```python
from build123d import *

# Parameters (mm, degrees)
F0_R     = 20
F0_R_2   = 1.5
F1_DEPTH = 4
F2_R     = 21.4
F2_R_2   = 20
F3_DEPTH = 1
F4_R     = 21.4
F4_R_2   = 20
F5_DEPTH = 1


with BuildPart() as f1:
    # F0 (on Top) → F1 (new body)
    with BuildSketch(Plane.XY):
        Circle(F0_R)
        Circle(F0_R_2, mode=Mode.SUBTRACT)
    extrude(amount=F1_DEPTH)

    # F2 (on face) → F3 (join)
    with BuildSketch(Plane.XY.offset(4)):
        Circle(F2_R)
        Circle(F2_R_2, mode=Mode.SUBTRACT)
    extrude(amount=-F3_DEPTH)

    # F4 (on face) → F5 (join)
    with BuildSketch(Plane(origin=(0, 0, 0), x_dir=(1, 0, 0), z_dir=(0, 0, -1))):
        Circle(F4_R)
        Circle(F4_R_2, mode=Mode.SUBTRACT)
    extrude(amount=-F5_DEPTH)


solid = f1.part
```
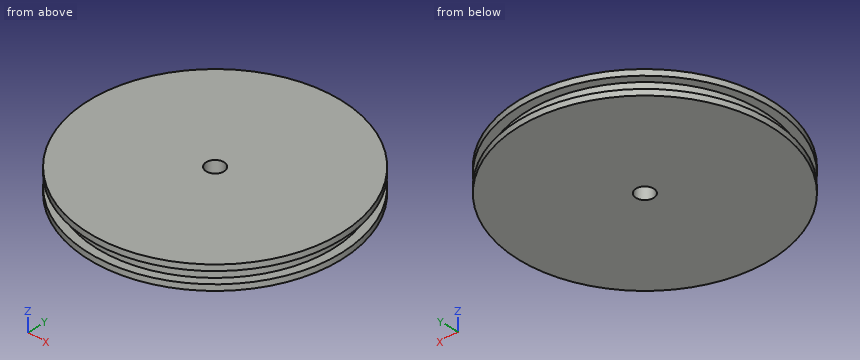
Input: part model. Units: mm. Frame: model coordinates. Give positions to 0.01 mm unless a question says otherwise; leave off trailing zeros. Order: outer loops, then holes, each group sorted by start corner. A loop starts at its lowest first (then second) coordinate and runs counter-clockwise, first axis right, second up.
1. Cut plane A-A (y = 0). Return loops of the section in (x, z), and give its area (3 significant figures).
Computed:
outline: (-21.4, 0) - (-1.5, 0) - (-1.5, 4) - (-21.4, 4) - (-21.4, 3) - (-20, 3) - (-20, 1) - (-21.4, 1) - close; (1.5, 0) - (21.4, 0) - (21.4, 1) - (20, 1) - (20, 3) - (21.4, 3) - (21.4, 4) - (1.5, 4) - close
area: 154 mm2
2. Cut plane C-C (x = -12.5). Return loops of the section in (y, z), and give its area (3 significant figures).
Computed:
outline: (-17.37, 0) - (17.37, 0) - (17.37, 1) - (15.61, 1) - (15.61, 3) - (17.37, 3) - (17.37, 4) - (-17.37, 4) - (-17.37, 3) - (-15.61, 3) - (-15.61, 1) - (-17.37, 1) - close
area: 132 mm2
3. Pin query (flat end, axial travel): pin 1 Ø13 at (x, y) = (-7, -1.5) entering from -Z; pin 2 Ø2 at (y, z) = (9.5, 2.5) entering from +X; pin 3 Ø1.5 at (y, z) = (-5, 2) entering from -X; pin 4 Ø1 at (x, z) = (-15.5, 3) entering from +Y. Return the tip coordinate at first contact, or that it passes through.
Computed:
pin 1: stops at z = 0
pin 2: stops at x = 19.58
pin 3: stops at x = -19.54
pin 4: stops at y = 15.26
4. Line query: probe 1 along Y at (x, z) = (0, 2); probe 2 along Z at (x, y) = (15, -14); probe 3 along Y at (x, z) = (9, 0.9). Output: solid intervals per line, ascending.
Computed:
probe 1: y = -20 to -1.5, 1.5 to 20
probe 2: z = 0 to 1, 3 to 4
probe 3: y = -19.42 to 19.42
5. Cut plane D-D (y = -10). Return loops of the section in (x, z).
Computed:
outline: (-18.92, 0) - (18.92, 0) - (18.92, 1) - (17.32, 1) - (17.32, 3) - (18.92, 3) - (18.92, 4) - (-18.92, 4) - (-18.92, 3) - (-17.32, 3) - (-17.32, 1) - (-18.92, 1) - close
